```python
from build123d import *

# Parameters (mm, degrees)
SKETCH_1_W          = 30
SKETCH_1_H          = 40
EXTRUDE_1_DEPTH     = 3
SKETCH_2_W          = 30
SKETCH_2_H          = 3
EXTRUDE_2_DEPTH     = 17
SKETCH_5_W          = 37
SKETCH_5_H          = 3
CUT_EXTRUDE_3_DEPTH = 10
SKETCH_6_W          = 20
SKETCH_6_H          = 3
CUT_EXTRUDE_4_DEPTH = 10
SKETCH_7_W          = 20
SKETCH_7_H          = 17
CUT_EXTRUDE_5_DEPTH = 1
SKETCH_8_W          = 20
SKETCH_8_H          = 28
CUT_EXTRUDE_6_DEPTH = 1
SKETCH_10_R         = 1.5
CUT_EXTRUDE_7_DEPTH = 10
SKETCH_11_R         = 1.5
CUT_EXTRUDE_8_DEPTH = 10


with BuildPart() as part:
    # 草图1 → 凸台-拉伸1 (new body)
    with BuildSketch(Plane(origin=(0, 0, 0), x_dir=(1, 0, 0), z_dir=(0, 1, 0))):
        with Locations((-6.335311573, -13.086053412)):
            Rectangle(SKETCH_1_W, SKETCH_1_H)
    extrude(amount=EXTRUDE_1_DEPTH)

    # 草图2 → 凸台-拉伸2 (add)
    with BuildSketch(Plane(origin=(0, 3, 0), x_dir=(1, 0, 0), z_dir=(0, 1, 0))):
        with Locations((-6.335311573, 5.413946588)):
            Rectangle(SKETCH_2_W, SKETCH_2_H)
    extrude(amount=EXTRUDE_2_DEPTH)

    # 草图5 → 切除-拉伸3 (cut)
    with BuildSketch(Plane(origin=(8.664688427, 0, 0), x_dir=(0, 0, -1), z_dir=(1, 0, 0))):
        Polygon((6.913946588, 20), (3.913946588, 20), (3.913946588, 3), (3.913946588, 0), (6.913946588, 0), align=None)
        with Locations((-14.586053412, 1.5)):
            Rectangle(SKETCH_5_W, SKETCH_5_H)
    extrude(amount=-CUT_EXTRUDE_3_DEPTH, mode=Mode.SUBTRACT)

    # 草图6 → 切除-拉伸4 (cut)
    with BuildSketch(Plane.XY.offset(33.086053412)):
        with Locations((-11.335311573, 1.5)):
            Rectangle(SKETCH_6_W, SKETCH_6_H)
    extrude(amount=-CUT_EXTRUDE_4_DEPTH, mode=Mode.SUBTRACT)

    # 草图7 → 切除-拉伸5 (cut)
    with BuildSketch(Plane.XY.offset(-3.913946588)):
        with Locations((-11.335311573, 11.5)):
            Rectangle(SKETCH_7_W, SKETCH_7_H)
    extrude(amount=-CUT_EXTRUDE_5_DEPTH, mode=Mode.SUBTRACT)

    # 草图8 → 切除-拉伸6 (cut)
    with BuildSketch(Plane(origin=(0, 3, 0), x_dir=(1, 0, 0), z_dir=(0, 1, 0))):
        with Locations((-11.335311573, -9.086053412)):
            Rectangle(SKETCH_8_W, SKETCH_8_H)
    extrude(amount=-CUT_EXTRUDE_6_DEPTH, mode=Mode.SUBTRACT)

    # 草图10 → 切除-拉伸7 (cut)
    with BuildSketch(Plane.XZ):
        with Locations((-8.335311573, 7.086053412)):
            Circle(SKETCH_10_R)
        with Locations((-8.335311573, 19.086053412)):
            Circle(SKETCH_10_R)
        with Locations((-18.335311573, 7.086053412)):
            Circle(SKETCH_10_R)
        with Locations((-18.335311573, 19.086053412)):
            Circle(SKETCH_10_R)
    extrude(amount=-CUT_EXTRUDE_7_DEPTH, mode=Mode.SUBTRACT)

    # 草图11 → 切除-拉伸8 (cut)
    with BuildSketch(Plane.XY.offset(-4.913946588)):
        with Locations((-5.335311573, 6)):
            Circle(SKETCH_11_R)
        with Locations((-17.335311573, 6)):
            Circle(SKETCH_11_R)
        with Locations((-5.335311573, 16)):
            Circle(SKETCH_11_R)
        with Locations((-17.335311573, 16)):
            Circle(SKETCH_11_R)
    extrude(amount=-CUT_EXTRUDE_8_DEPTH, mode=Mode.SUBTRACT)


solid = part.part
```
Geometry check sheet. Reference: the model listing, model coordinates, mm. A direction names the side the tool comes from. Round coordinates to 2 decimals unless told otherwise and drop trailing zeros. Loops run counter-clockwise (first coordinate to the right, second up) from the corner with the lowest first, then second, coordinate; pieces in that order, holes last. Notation, with made-up numbers: M 11,37.5 L 44,37.5 A15 cw 44,47.5 Z; hole C 41,-5.75 d9. An arc over 180 degrees is marked long. Return JSON: item names as keys, results as strings. Group by question number.
(1) Section check D-D, the plane x = -12. Enter the section's corners in (y, z).
(2) Mould release check, pull along Y, two halves, no side actions. Record for faces 3 (the face through (-11, 0, 8)), 4 (the face through (-3.95, 5.425, -5.9)), 5 (the face through (-11, 10, -6.914)): pulls with the +Y half, pulls with the -Y half, needs draft (parallel to the pull), parting line crosses it, or undercut.
(3) Set-up check for faces 1 (the face through (-16.95, 0.99, 18.51)), 2 (the face through (-11, 2, 9)): record each of +Z, -Z, +X, -X, +Y, -Y from which the full face is reachable in a straight line by a thin tool's end or side.
(4) Section check A-A, the plane y = 6. Enter the section's corners in (x, z), and give its area (3 significant figures).
(5) Section check B-B, the plane x = -6.25. Enter the section's corners in (y, z), and give its area (3 significant figures).
(6) Go/stop test with flat-tipped pins: pin 1 (2.5 mm diameter, centred on x = -18.34, z = 7.09, fed in from +Y); pin 2 (4 mm diameter, centred on x = -10.5, z = 8.5, fed in from +Y); pin 3 (8 mm diameter, centred on x = -10.5, y = 16, fed in from +Z). Record where each tip stops, or that it passes through.
(7) Section check C-C, the plane z = 6. Enter the section's corners in (x, y).
(8) Scan lines: line 1 along Y through (x, z) = (-17.25, -5.5); line 2 along Y through (x, z) = (-6, -0.75); line 3 along Z through (x, y) = (-13, 6.75). Record each from-to range of solid material in increasing order. Write a range as [from, to].
Data:
{
 "1": {"outline": "M 0,-6.91 L 20,-6.91 L 20,-4.91 L 2,-4.91 L 2,23.09 L 0,23.09 Z"},
 "2": {"face 3": "pulls with the -Y half", "face 4": "undercut", "face 5": "needs draft"},
 "3": {"face 1": "+Y, -Y", "face 2": "+Z, +X, -X, +Y"},
 "4": {"outline": "M -21.34,-6.91 L -18.84,-6.91 L -18.84,-4.91 L -21.34,-4.91 Z; M -15.84,-6.91 L -6.84,-6.91 L -6.84,-4.91 L -15.84,-4.91 Z; M -3.84,-6.91 L -1.34,-6.91 L -1.34,-4.91 L -3.84,-4.91 Z", "area": "28.0 mm²"},
 "5": {"outline": "M 0,-6.91 L 4.81,-6.91 L 4.81,-4.91 L 2,-4.91 L 2,23.09 L 0,23.09 Z; M 7.19,-6.91 L 14.81,-6.91 L 14.81,-4.91 L 7.19,-4.91 Z; M 17.19,-6.91 L 20,-6.91 L 20,-4.91 L 17.19,-4.91 Z", "area": "86.5 mm²"},
 "6": {"pin 1": "through", "pin 2": "y = 2", "pin 3": "z = -4.91"},
 "7": {"outline": "M -21.34,0 L -19.37,0 L -19.37,2 L -21.34,2 Z; M -17.3,0 L -9.37,0 L -9.37,2 L -17.3,2 Z; M -7.3,0 L -1.34,0 L -1.34,2 L -7.3,2 Z"},
 "8": {"line 1": "[0, 4.5], [7.5, 14.5], [17.5, 20]", "line 2": "[0, 2]", "line 3": "[-6.91, -4.91]"}
}
